Answer from the drawing. Dimensions are ordinates in mm from the lowest x, y and z of the part. Round coordinates to 2 decimals unless told otherwise and drop trailing zeros. Order: outer loops, then holes, each group sorted by start corner. A loop starts at its lowest first (then second) coordinate and runs counter-clockwise, first axis right, second up.
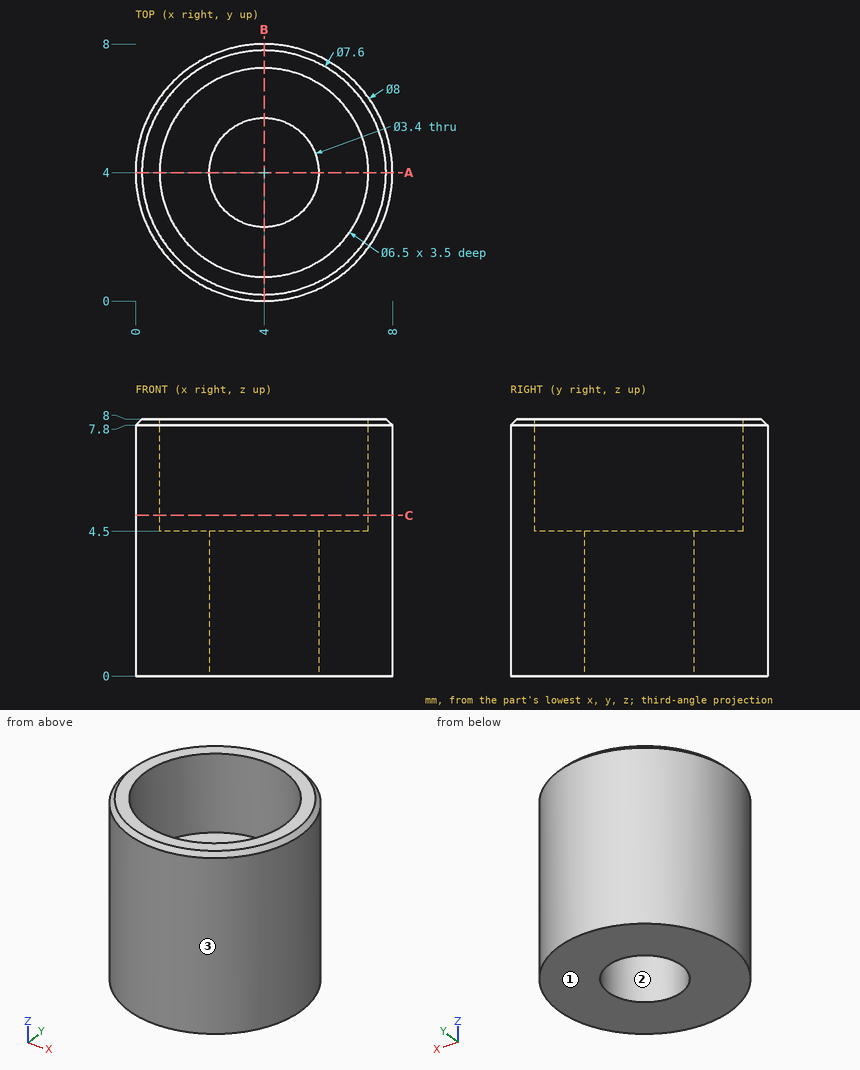
Q1. Flat-ended cylindrical pins translate along their axes: pin 1 (2 mm diameter, centred on x = 5, z = 3, fed in from +Y); pin 2 (2 mm diameter, centred on x = 2.5, y = 4, fed in from +Z); pin 3 (2 mm diameter, centred on y = 1.5, z = 1.5, fed in from +X); pin 4 (1 mm diameter, centred on y = 7, z = 4.5, fed in from -X). Find the tip coordinate at first contact, or state that the pin passes through.
Outcome:
pin 1: stops at y = 8
pin 2: stops at z = 4.5
pin 3: stops at x = 7.71
pin 4: stops at x = 0.88
Q2. Straight lines are drawn through the part: probe 1 along Y at (x, z) = (4, 7.05); probe 2 along Y at (x, z) = (4, 3.5); probe 3 along Z at (x, y) = (1.25, 2.5). For each, find the intervals that lie inside material, in ascending order.
Outcome:
probe 1: y = 0 to 0.75, 7.25 to 8
probe 2: y = 0 to 2.3, 5.7 to 8
probe 3: z = 0 to 4.5
Q3. A cutting plane is placed at A-A, the plane y = 4. Give the vertices of the cut face in (x, z).
Outcome:
outline: (0, 0) - (2.3, 0) - (2.3, 4.5) - (0.75, 4.5) - (0.75, 8) - (0.2, 8) - (0, 7.8) - close; (5.7, 0) - (8, 0) - (8, 7.8) - (7.8, 8) - (7.25, 8) - (7.25, 4.5) - (5.7, 4.5) - close
Q4. A cutting plane is placed at C-C, the plane z = 5. Give the vertices of the cut face in (x, y), plus the area to 3 significant figures.
Outcome:
outline: circle Ø8 at (4, 4); hole circle Ø6.5 at (4, 4)
area: 17.1 mm2
Q5. For a pull along X with two mould halves and no side action, classify the marked faces 1, 2 and 3 as released by +X, released by -X, zero draft, split by the parting line, or undercut.
Outcome:
face 1: zero draft
face 2: undercut
face 3: split by the parting line
